Part model, mm, in its own coordinate system. A direction names the side the tool comes from. Round coordinates to 2 decimals unless told otherwise and drop trailing zeros. Loops run counter-clockwise (first coordinate to the right, second up) from the corner with the lowest first, then second, coordinate; pieces in that order, holes last. Notation, with made-up numbers: (29.25, 23) -> (55.25, 23) arc R27 cw to (55.25, 44) -> close; hole circle Ø10 at (89, -32). An arc over 180 degrees is marked (long way). Use a Markdown table: item, result. Add a question column.
Item 1: Cut at A-A, the plane x = -6. List the corners of the cut face in (y, z), plus the area to 3 significant figures.
Item 2: Flat gauge pins, fed straight in: pin 1 (5 mm diameter, centred on x = 25.5, y = -5, fed in from +Z); pin 2 (5 mm diameter, centred on x = 18.5, y = 6.5, fed in from +Z); pin 3 (3.5 mm diameter, centred on x = -72.5, y = 13.5, fed in from +Z); pin 4 (3 mm diameter, centred on x = 72.5, y = -11.5, fed in from -Z). Where does each tip first touch, or does it go through?
Item 3: Probe line 1 (Y direction, x = 72.5, z = -56.2); line 2 (Y direction, x = -5.5, z = 6); line 3 (Z direction, x = 5, y = -11.75). List the from-to ranges inside material, lowest first. Write a range as [from, to].
Item 4: Which spindle directions (+Z, -Z, +X, -X, +Y, -Y) get a long thin tool onto all of the face, cutting with end or side? Do faces 1 (the face through (-1, -14, -56)), 2 (the face through (1, 2, 6)), 3 (the face through (1, -12, -55)). Say none if no direction does.
Item 5: Cut at C-C, the plane y = 9.25. List the corners of the cut face in (x, z), plus the area to 3 significant figures.
Item 6: Cut at B-B, the plane z = -25. List the corners of the cut face in (x, y).
Autodesk Inventor part; units mm, degrees
ref_plane "YZ Plane" through (0, 0, 0) normal (1, 0, 0) x (0, 1, 0)
ref_plane "XZ Plane" through (0, 0, 0) normal (0, 1, 0) x (-1, 0, 0)
ref_plane "XY Plane" through (0, 0, 0) normal (0, 0, 1) x (1, 0, 0)
sketch "Sketch1" plane through (0, 0, 0) normal (0, 1, 0) x (-1, 0, 0)
  line L0 (75, 55) -> (-75, 55)
  line L1 (-75, 55) -> (-75, -55)
  line L2 (-75, -55) -> (75, -55)
  line L3 (75, -55) -> (75, 55)
  line L4 (75, 55) -> (-75, -55) construction
  line L5 (-75, 55) -> (75, -55) construction
  point P0 (0, 0)
  dimension "d0" = 150
  dimension "d1" = 110
extrude "Extrusion1" add sketch "Sketch1" along normal blind 2
sketch "Sketch2" plane through (75, 0, -55) normal (0, 0, -1) x (-1, 0, 0)
  line L0 (0, 0) -> (150, 0)
  line L1 (150, 0) -> (150, 2)
  line L2 (0, 2) -> (150, 2)
  line L3 (0, 0) -> (0, 2)
  line L4 (0, 0) -> (0, 2) construction
  line L5 (0, 0) -> (150, 2) construction
  line L6 (150, 0) -> (0, 0) construction
  line L7 (150, 0) -> (0, 2) construction
  line L8 (150, -14) -> (0, -14)
  line L9 (0, -14) -> (0, 16)
  line L10 (0, 16) -> (150, 16)
  line L11 (150, 16) -> (150, -14)
  line L12 (150, -14) -> (0, 16) construction
  line L13 (0, -14) -> (150, 16) construction
  point P0 (75, 0)
  point P1 (75, 1)
  dimension "d4" = 30
  dimension "d5" = 150
extrude "Extrusion2" add sketch "Sketch2" along normal blind 3
fillet "Fillet1" radius 10 2 edges at (0, 0, -55) (0, 2, -55)
sketch "Sketch3" plane through (0, 0, 0) normal (0, -1, 0) x (1, 0, 0)
  line L0 (0, 0) -> (0, 5)
  line L1 (0, 0) -> (5, 0) construction
  line L2 (-50, 55) -> (50, 55)
  line L3 (50, 55) -> (50, -45)
  line L4 (50, -45) -> (-50, -45)
  line L5 (-50, -45) -> (-50, 55)
  line L6 (-50, 55) -> (50, -45) construction
  line L7 (50, 55) -> (-50, -45) construction
  line L8 (-50, 55) -> (-53, 55)
  line L9 (-53, 55) -> (-53, 50)
  line L10 (-53, 50) -> (-50, 50)
  line L11 (-50, 50) -> (-50, 55)
  line L12 (50, 55) -> (53, 55)
  line L13 (53, 55) -> (53, 50)
  line L14 (53, 50) -> (50, 50)
  line L15 (50, 50) -> (50, 55)
  dimension "d9" = 5
  dimension "d10" = 90
  dimension "d11" = 100
  dimension "d12" = 100
  dimension "d13" = 3
  dimension "d14" = 5
  dimension "d15" = 3
  dimension "d16" = 5
extrude "Extrusion3" cut sketch "Sketch3" against normal up to surface (2 mm away) contours L5 L10 L9 L8 | L12 L13 L14 L3
sketch "Sketch4" plane through (75, 0, -58) normal (0, 0, -1) x (-1, 0, 0)
  line L0 (75, 0) -> (147.5, 0)
  line L1 (0, 0) -> (150, 0)
  line L2 (75, 0) -> (147.5, 0) construction
  line L3 (147.5, 0) -> (147.5, -11.5)
  line L4 (150, -10) -> (0, -10)
  circle A0 centre (147.5, -11.5) radius 1.35
  line L5 (75, 0) -> (75, -10)
  line L6 (75, 0) -> (85, 0) construction
  circle A1 centre (147.5, 13.5) radius 1.35
  circle A2 centre (2.5, -11.5) radius 1.35
  circle A3 centre (2.5, 13.5) radius 1.35
  line L7 (150, 2) -> (0, 2)
  line L8 (75, 0) -> (75, 1)
  line L9 (75, 0) -> (76, 0) construction
  dimension "d19" = 72.5
  dimension "d20" = 0
  dimension "d21" = 11.5
  dimension "d22" = 90
  dimension "d23" = 2.7
  dimension "d24" = 10
  dimension "d25" = 90
  dimension "d28" = 25
  dimension "d31" = 145
  dimension "d34" = 1
  dimension "d35" = 90
extrude "Extrusion4" cut sketch "Sketch4" against normal up to surface (3 mm away) contours A0 | A1 | A2 | A3
properties part number "apriltag_body"
A:
| question | item | result |
|---|---|---|
| 1 | outline | (-14, -58) -> (16, -58) -> (16, -55) -> (12, -55) arc R10 cw to (2, -45) -> (2, 55) -> (0, 55) -> (0, -45) arc R10 cw to (-10, -55) -> (-14, -55) -> close |
| 1 | area | 353 mm^2 |
| 2 | pin 1 | stops at z = -51.61 |
| 2 | pin 2 | stops at z = -51 |
| 2 | pin 3 | stops at z = -55 |
| 2 | pin 4 | stops at z = -58 |
| 3 | line 1 | y = [-14, -12.85], [-10.15, 12.15], [14.85, 16] |
| 3 | line 2 | y = [0, 2] |
| 3 | line 3 | z = [-58, -55] |
| 4 | face 1 | +Z, -Z, +X, -X, -Y |
| 4 | face 2 | +Z, +X, -X, +Y |
| 4 | face 3 | +Z, +X, -X, -Y |
| 5 | outline | (-75, -58) -> (75, -58) -> (75, -54.61) -> (-75, -54.61) -> close |
| 5 | area | 508 mm^2 |
| 6 | outline | (-75, 0) -> (75, 0) -> (75, 2) -> (-75, 2) -> close |
